Design review of the part shown in the three views and the two pictorial views. Dimensions are in mm from the part's minimum x, y and z. Coordinates: 2 decimals unless noted, no trailing zeros. Loops run counter-clockwise (first coordinate to the right, second up) from the corner with the lowest first, then second, coordinate; pieces in that order, holes last. Notation, with made-up numbers: (78, -1.75) -> (108, -1.75) arc R23 cw to (108, 30.25) -> close; hole circle Ø11 at (10, 28). An arc over 180 degrees is marked (long way). Answer in a Markdown table with one row per item.
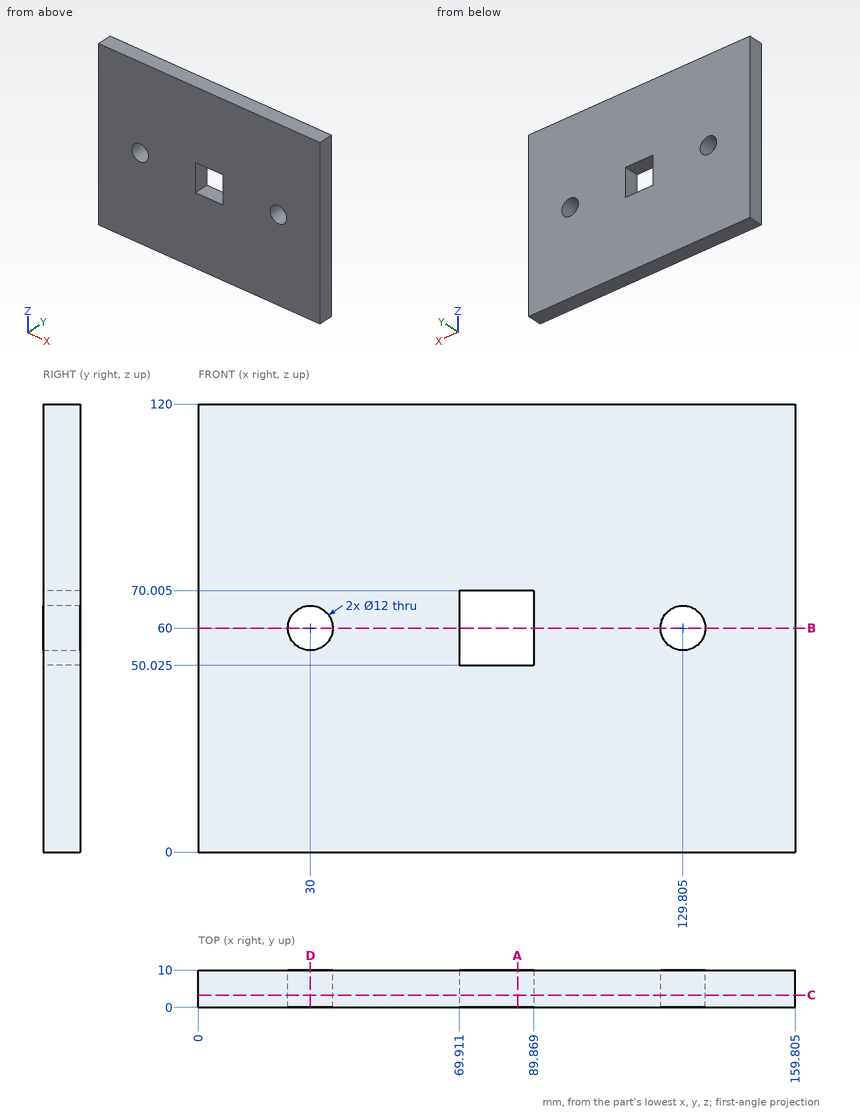
(1) For pin 1 (7 mm diameter, centred on x = 30, z = 60, fed in from +Y), flat-tipped, find the tip position at first contact; note if it passes through.
Evaluation:
| item | result |
|---|---|
| pin 1 | passes through |
(2) To check wall thickness, follow probe 1 along X at (y, z) = (6, 60) (1 decimal); probe 2 along Z at (x, y) = (30, 5.5); probe 3 along X at (y, z) = (7.5, 53.5) (1 decimal). State the ranges of each line that lie inside material, in increasing order.
Evaluation:
| item | result |
|---|---|
| probe 1 | x = 0 to 24, 36 to 69.9, 89.9 to 123.8, 135.8 to 159.8 |
| probe 2 | z = 0 to 54, 66 to 120 |
| probe 3 | x = 0 to 69.9, 89.9 to 159.8 |
(3) Take a section at B-B on z = 60. Give the boundary of the cut face in (x, y) (1 decimal).
Evaluation:
| item | result |
|---|---|
| outline | (0, 0) -> (24, 0) -> (24, 10) -> (0, 10) -> close; (36, 0) -> (69.9, 0) -> (69.9, 10) -> (36, 10) -> close; (89.9, 0) -> (123.8, 0) -> (123.8, 10) -> (89.9, 10) -> close; (135.8, 0) -> (159.8, 0) -> (159.8, 10) -> (135.8, 10) -> close |
(4) Take a section at D-D on x = 30. Give the boundary of the cut face in (y, z).
Evaluation:
| item | result |
|---|---|
| outline | (0, 0) -> (10, 0) -> (10, 54) -> (0, 54) -> close; (0, 66) -> (10, 66) -> (10, 120) -> (0, 120) -> close |
(5) Take a section at C-C on y = 3.25. Give the boundary of the cut face in (x, z) (1 decimal).
Evaluation:
| item | result |
|---|---|
| outline | (0, 0) -> (159.8, 0) -> (159.8, 120) -> (0, 120) -> close; hole circle Ø12 at (30, 60); hole (69.9, 50) -> (89.9, 50) -> (89.9, 70) -> (69.9, 70) -> close; hole circle Ø12 at (129.8, 60) |
(6) Take a section at A-A on x = 85.5. Give the boundary of the cut face in (y, z) (1 decimal), and give its area (3 significant figures).
Evaluation:
| item | result |
|---|---|
| outline | (0, 0) -> (10, 0) -> (10, 50) -> (0, 50) -> close; (0, 70) -> (10, 70) -> (10, 120) -> (0, 120) -> close |
| area | 1,000 mm² |
